For this review, take the finished solid that the model builds, in its own axes (mm). Face numbers are marked on the shaded views. A direction names the side the tool comes from. Give positions to 0.01 mm unless a question says otherwise; leave off trailing zeros. Write each loop counter-clockwise with the first axis right and the second up, starting at its lowest first coordinate (ties: lowest second). Pieces come first, ordered by that corner, then holes.
Q1. Machinability: for the marked faces 1 and 2, which of the approach directions +Z, -Z, +X, -X, +Y, -Y give a long, thin tool a straight path to every point of the face, cutting with its end or side? Answer none if there is none.
Q2. Mouldability with a two-part tool opening along X and no side actions: class the marked faces 3 and 4 as released by +X, released by -X, zero draft, split by the parting line, or undercut.
Q3. We need section A-A (z = -6.5). Write out the cut boundary in (x, y), then the cut area to 3 significant figures.
Q4. For line 1 (X direction, y = 0.1, z = -11.25); line 2 (X direction, y = 1.35, z = -1.5); line 3 (Y direction, x = -0.1, z = -2), list the stretches that pass through material, from the lowest coordinate up.
Q5. Insertion check: P1, Ø3, axis at x = 1, z = -4, coming from the +Y side; P2, Ø3, axis at x = -1.5, y = -2, coming from the -Z side; P3, Ø1.4, axis at y = 0.5, z = -1.5, coming from the -X side; P4, Ø2, axis at x = -2, z = -1.5, coming from the -Y side. Each pin has a flat end and moves straight along its axis. Give the tip position at first contact, or say it passes through.
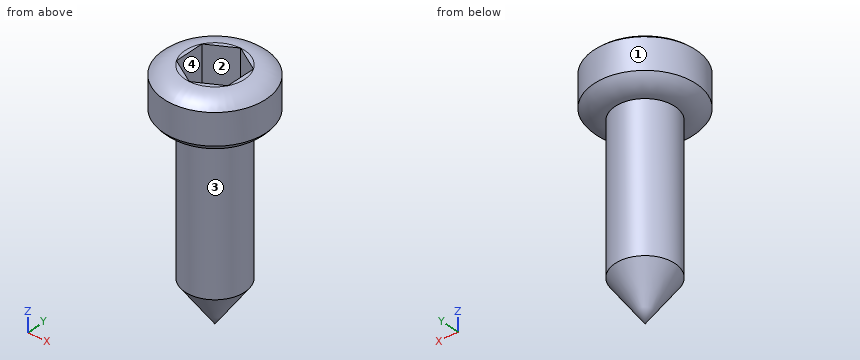
```python
from build123d import *

# Parameters (mm, degrees)
CUT_EXTRUDE1_DEPTH = 2.5


with BuildPart() as part:
    # Sketch1 → Revolve1 (revolve)
    with BuildSketch(Plane(origin=(0, 0, 0), x_dir=(0, 0, -1), z_dir=(1, 0, 0)), mode=Mode.PRIVATE) as revolve1_sk:
        with BuildLine():
            Line((0, 0), (14, 0))
            Line((14, 0), (11.5, 1.75))
            Line((11.5, 1.75), (3.017689414, 1.75))
            ThreePointArc((3.017689414, 1.75), (2.839380432, 2.459318583), (2.346845612, 3))
            Line((2.346845612, 3), (0.527441756, 3))
            ThreePointArc((0.527441756, 3), (0.137258951, 2.428361041), (0, 1.75))
            Line((0, 1.75), (0, 0))
        make_face()
    revolve(revolve1_sk.sketch.rotate(Axis((0, 0, 0), (0, 0, -1)), 90), axis=Axis((0, 0, 0), (0, 0, -1)))

    # Sketch7 → Cut-Extrude1 (cut)
    with BuildSketch(Plane.XY):
        Polygon((-1.515544457, 0.875), (-1.515544457, -0.875), (0, -1.75), (1.515544457, -0.875), (1.515544457, 0.875), (0, 1.75), align=None)
    extrude(amount=-CUT_EXTRUDE1_DEPTH, mode=Mode.SUBTRACT)


solid = part.part
```
Computed:
1. face 1: +Z, -Z
1. face 2: +Z
2. face 3: split by the parting line
2. face 4: undercut
3. outline: circle Ø3.5 at (0, 0)
3. area: 9.62 mm2
4. line 1: x = -1.75 to 1.75
4. line 2: x = -2.68 to -0.69, 0.69 to 2.68
4. line 3: y = -3 to -1.69, 1.69 to 3
5. P1: stops at y = 2.77
5. P2: stops at z = -12.57
5. P3: stops at x = -3
5. P4: stops at y = -2.83
